Verification items for the finished model (mm, model axes). A direction names the side the tool comes from. Coordinates: 2 decimals unless noted, no trailing zeros. Order: outer loops, then holes, each group sorted by start corner. A loop starts at its lowest first (then second) coordinate and runs counter-clockwise, first axis right, second up. Notation, with made-up numbers: M -4,-12 L 26,-12 A23 cw 26,14 Z; hole C -19,32 d8. An arc over 180 degrees is marked long. Answer as a JSON object with one key per item and string values. Group by question number.
(1) Material ranges on line 1 (Z direction, x = -2, y = 5.5); line 2 (Y direction, x = 3.25, z = 20); line 3 (X direction, y = -4.5, z = 23.5), recorded low to high.
(2) Cross-section at A-A (x = 0). Enter the section's corners in (y, z), plus the area to 3 significant figures.
(3) Access from +Z, -Z, +X, -X, +Y, -Y to the whole of each face (thin tool, end or side, straight path). Record for faces 1 (the face through (-6.09, -3.45, 61.48)), 2 (the face through (-1.08, -4.88, 30.09)).
(4) Cross-section at B-B (z = 52.5). Enter the section's corners in (x, y).
(5) Gauge pin test, flat ends, axial feed: pin 1 Ø4 at (y, z) = (4, 15.5) entering from +X; pin 2 Ø5 at (x, z) = (5.5, 54.5) entering from -Y. Record the tip position at first contact, or that the pin passes through.
from build123d import *

# Parameters (mm, degrees)
F0_R     = 5
F1_DEPTH = 60
F2_SIZE2 = 1
F2_SIZE  = 1
F4_DEPTH = 3


with BuildPart() as f1:
    # F0 (on Top) → F1 (new body)
    with BuildSketch(Plane.XY):
        Circle(F0_R)
    extrude(amount=F1_DEPTH)

    # F2
    f2_edges = [f1.edges().sort_by_distance(p)[0] for p in [
        (-5, 0, 0),
    ]]
    chamfer(f2_edges, length=F2_SIZE, length2=F2_SIZE2)

    # F3 (on face) → F4 (join)
    with BuildSketch(Plane.XY.offset(60)):
        Polygon((8.082904, 0), (4.041452, 7), (-4.041452, 7), (-8.082904, 0), (-4.041452, -7), (4.041452, -7), align=None)
    extrude(amount=F4_DEPTH)


solid = f1.part
Taken from the geometry:
{
 "1": {"line 1": "z = 60 to 63", "line 2": "y = -3.8 to 3.8", "line 3": "x = -2.18 to 2.18"},
 "2": {"outline": "M -7,60 L -5,60 L -5,1 L -4,0 L 4,0 L 5,1 L 5,60 L 7,60 L 7,63 L -7,63 Z", "area": "641 mm²"},
 "3": {"face 1": "+Z, -Z, -X, -Y", "face 2": "-Z"},
 "4": {"outline": "C 0,0 d10"},
 "5": {"pin 1": "stops at x = 4.58", "pin 2": "stops at y = -4"}
}
